```python
from build123d import *

# Parameters (mm, degrees)
SKETCH4_W           = 13.18
SKETCH4_H           = 14.85
BOSS_EXTRUDE2_DEPTH = 10
CUT_EXTRUDE1_DEPTH  = 5


with BuildPart() as part:
    # Sketch4 → Boss-Extrude2 (new body)
    with BuildSketch(Plane(origin=(0, 0, 0), x_dir=(1, 0, 0), z_dir=(0, 1, 0))):
        with Locations((-115.17, 78.265)):
            Rectangle(SKETCH4_W, SKETCH4_H)
    extrude(amount=BOSS_EXTRUDE2_DEPTH)

    # Sketch5 → Cut-Extrude1 (cut)
    with BuildSketch(Plane.XZ):
        with BuildLine():
            ThreePointArc((-120.17, -78.265), (-115.17, -83.265), (-110.17, -78.265))
            Line((-110.17, -78.265), (-120.17, -78.265))
        make_face()
        with BuildLine():
            Line((-120.17, -78.265), (-110.17, -78.265))
            ThreePointArc((-110.17, -78.265), (-115.17, -73.265), (-120.17, -78.265))
        make_face()
    extrude(amount=-CUT_EXTRUDE1_DEPTH, mode=Mode.SUBTRACT)


solid = part.part
```
Check sheet for the modelled part. Datum: model origin and axes. Units: mm. A direction names the side the tool comes from. Give positions to 0.01 mm unless a question says otherwise; leave off trailing zeros. Write each loop counter-clockwise with the first axis right and the second up, starting at its lowest first coordinate (ties: lowest second). Pieces come first, ordered by that corner, then holes. Notation, with made-up numbers: (1, 31.25) - (39, 31.25) arc R29 ccw to (39, 52.25) - close; hole circle Ø8 at (-38.5, 49.25). An arc over 180 degrees is marked (long way). Answer as a JSON object with one key per item and string values. Group by question number.
1) Sectioned sample at C-C (z = -80). Record the cut outline in (x, y).
2) Sectioned sample at B-B (x = -115.17). Record the cut outline in (y, z) (3 decimals).
3) Depth check by flat-ended pin: P1, Ø3, axis at x = -117.5, z = -78.5, coming from the -Y side. Enter the tip coordinate at first touch or a pass-through.
4) Access from +Z, -Z, +X, -X, +Y, -Y to the whole of each face (thin tool, end or side, straight path). Record for faces 1 (the face through (-116.7, 0, -83.3)), 2 (the face through (-115, 5, -78)).
5) Release check for a two-part mould opening along X. For faces 3 (the face through (-120.165, 2.465, -78.045)), 4 (the face through (-115, 10, -78)), 5 (the face through (-108.58, 5, -78)) record: pulls with the +X half, pulls with the -X half, needs draft (parallel to the pull), parting line crosses it, or undercut.
6) Sectioned sample at A-A (y = 3.5). Record the cut outline in (x, z) (3 decimals).
7) Thickness scan on probe 1 along Z at (x, y) = (-115.17, 3.35) (3 decimals); probe 2 along Y at (x, z) = (-114.25, -73.5); probe 3 along X at (y, z) = (3.5, -77.75). Record the ranges inside material, lowest first. Write a range as from..to.
Geometry results:
{
 "1": {"outline": "(-121.76, 0) - (-119.86, 0) - (-119.86, 5) - (-110.48, 5) - (-110.48, 0) - (-108.58, 0) - (-108.58, 10) - (-121.76, 10) - close"},
 "2": {"outline": "(0, -85.69) - (10, -85.69) - (10, -70.84) - (0, -70.84) - (0, -73.265) - (5, -73.265) - (5, -83.265) - (0, -83.265) - close"},
 "3": {"P1": "stops at y = 5"},
 "4": {"face 1": "+Z, -Z, +X, -X, -Y", "face 2": "-Y"},
 "5": {"face 3": "undercut", "face 4": "needs draft", "face 5": "pulls with the +X half"},
 "6": {"outline": "(-121.76, -85.69) - (-108.58, -85.69) - (-108.58, -70.84) - (-121.76, -70.84) - close; hole circle Ø10 at (-115.17, -78.265)"},
 "7": {"probe 1": "z = -85.69..-83.265, -73.265..-70.84", "probe 2": "y = 5..10", "probe 3": "x = -121.76..-120.14, -110.2..-108.58"}
}
